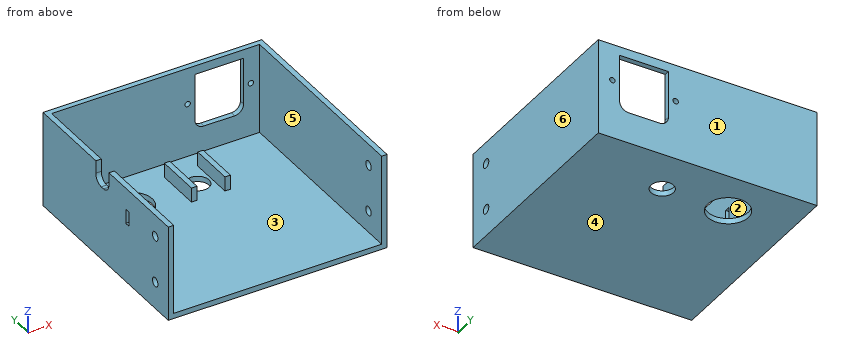
```python
from build123d import *

# Parameters (mm, degrees)
F0_W      = 121
F0_H      = 115
F1_DEPTH  = 3
F3_DEPTH  = 50
F4_R      = 2.5
F5_DEPTH  = 121.001
F6_R      = 11.25
F6_R_2    = 6.25
F7_DEPTH  = 25
F8_W      = 3
F8_H      = 25
F9_DEPTH  = 8
F10_R     = 1.5
F11_DEPTH = 25
F13_DEPTH = 25
F14_R     = 2.5
F14_W     = 3
F14_H     = 8
F15_DEPTH = 25


with BuildPart() as f1:
    # F0 (on Top) → F1 (new body)
    with BuildSketch(Plane.XY):
        with Locations((-4.051243, 22.351279)):
            Rectangle(F0_W, F0_H)
    extrude(amount=F1_DEPTH)

    # F2 (on face) → F3 (join)
    with BuildSketch(Plane.XY.offset(3)):
        Polygon((56.448757, 79.851279), (-64.551243, 79.851279), (-64.551243, -35.148721), (-61.551243, -35.148721), (-61.551243, 76.851279), (53.448757, 76.851279), (53.448757, -35.148721), (56.448757, -35.148721), align=None)
    extrude(amount=F3_DEPTH)

    # F4 (on face) → F5 (cut, through all)
    with BuildSketch(Plane(origin=(-64.551243, 0, 0), x_dir=(0, -1, 0), z_dir=(-1, 0, 0))):
        with Locations((23.148721, 15)):
            Circle(F4_R)
        with Locations((23.148721, 41)):
            Circle(F4_R)
    extrude(amount=-F5_DEPTH, mode=Mode.SUBTRACT)

    # F6 (on face) → F7 (cut)
    with BuildSketch(Plane(origin=(0, 0, 0), x_dir=(1, 0, 0), z_dir=(0, 0, -1))):
        with Locations((-30.708815, -54.351279)):
            Circle(F6_R)
        with Locations((5.693216, -54.351279)):
            Circle(F6_R_2)
    extrude(amount=-F7_DEPTH, mode=Mode.SUBTRACT)

    # F8 (on face) → F9 (join)
    with BuildSketch(Plane.XY.offset(3)):
        with Locations((-3.556784, 54.730202)):
            Rectangle(F8_W, F8_H)
        with Locations((14.943216, 54.730202)):
            Rectangle(F8_W, F8_H)
    extrude(amount=F9_DEPTH)

    # F10 (on face) → F11 (cut)
    with BuildSketch(Plane(origin=(0, 79.851279, 0), x_dir=(-1, 0, 0), z_dir=(0, 1, 0))):
        with BuildLine():
            ThreePointArc((-44.634731, 22.153023), (-43.170264, 18.617489), (-39.634731, 17.153023))
            Line((-39.634731, 17.153023), (-22.634731, 17.153023))
            ThreePointArc((-22.634731, 17.153023), (-19.099197, 18.617489), (-17.634731, 22.153023))
            Line((-17.634731, 22.153023), (-17.634731, 48.153023))
            Line((-17.634731, 48.153023), (-44.634731, 48.153023))
            Line((-44.634731, 48.153023), (-44.634731, 22.153023))
        make_face()
        with Locations((-13.634731, 32.653023)):
            Circle(F10_R)
        with Locations((-48.634731, 32.653023)):
            Circle(F10_R)
    extrude(amount=-F11_DEPTH, mode=Mode.SUBTRACT)

    # F12 (on face) → F13 (cut)
    with BuildSketch(Plane(origin=(-64.551243, 0, 0), x_dir=(0, -1, 0), z_dir=(-1, 0, 0))):
        with BuildLine():
            Line((-19.351279, 62.000753), (-31.351279, 62.000753))
            Line((-31.351279, 62.000753), (-31.351279, 46))
            ThreePointArc((-31.351279, 46), (-29.886813, 42.464466), (-26.351279, 41))
            Line((-26.351279, 41), (-24.351279, 41))
            ThreePointArc((-24.351279, 41), (-20.815745, 42.464466), (-19.351279, 46))
            Line((-19.351279, 46), (-19.351279, 62.000753))
        make_face()
    extrude(amount=-F13_DEPTH, mode=Mode.SUBTRACT)

    # F14 (on face) → F15 (cut)
    with BuildSketch(Plane(origin=(-64.551243, 0, 0), x_dir=(0, -1, 0), z_dir=(-1, 0, 0))):
        with Locations((23.148721, 41)):
            Circle(F14_R)
        with Locations((-2.351279, 37)):
            Rectangle(F14_W, F14_H)
    extrude(amount=-F15_DEPTH, mode=Mode.SUBTRACT)


solid = f1.part
```
Can you work these out from the model? Positions are in its coordinate system, mm. Face numbers are marked on the shaded views. A direction names the side the tool comes from. Coordinates: 2 decimals unless noted, no trailing zeros. Loops run counter-clockwise (first coordinate to the right, second up) from the corner with the lowest first, then second, coordinate; pieces in that order, holes last. Notation, with made-up numbers: M 76.25,23 L 123.25,23 A9 ccw 123.25,31 Z; hole C 31.5,51 d7. An arc over 180 degrees is marked long. Put each result on its own line as item: value. Start each with the question number.
(1) Will these pins go through, and if not, where does the flat tip stop? pin 1 Ø6 at (x, y) = (25.5, 54) entering from +Z; pin 2 Ø1.5 at (x, y) = (-4, 50.5) entering from +Z; pin 3 Ø3.5 at (x, z) = (-3.5, 7) entering from -Y; pin 4 Ø8 at (x, y) = (26.5, 44.5) entering from -Z.
(2) Imagine slicing it at C-C on y = 12.5. List the corners of the cut face in (x, z) for me.
(3) Which directions (+Z, -Z, +X, -X, +Y, -Y) give clear straight access to the entire face, cutting with the end or side of a thin tool? Please do the marked faces 1 and 2.
(4) Imagine slicing it at D-D on x = -7.5. List the corners of the cut face in (y, z) for me.
(5) We'd pull the mould along X, two halves only. Please class the marked faces 3, 4, 5 and 6: +X half, -X half, draft (parallel to the pull), parting line (faces both ways), or undercut.
(6) Imagine slicing it at B-B on x = 31. List the corners of the cut face in (y, z) for me.
(7) Imagine slicing it at A-A on z = 15. List the corners of the cut face in (x, y) for me, and give its area (4 significant figures).
(8) I need wall thicknesses on probe 1 along X at (y, z) = (-9, 24); probe 2 along Z at (x, y) = (-7, -1.5); probe 3 along Y at (x, z) = (45.5, 18). Which ranges of each line are inside material? Lowest first, please.
Worked answers:
1. pin 1: stops at z = 3
1. pin 2: stops at z = 11
1. pin 3: stops at y = 42.23
1. pin 4: stops at z = 0
2. outline: M -64.55,0 L 56.45,0 L 56.45,53 L 53.45,53 L 53.45,3 L -61.55,3 L -61.55,53 L -64.55,53 Z
3. face 1: +Z, -Z, +X, -X, +Y
3. face 2: +Z, -Y
4. outline: M -35.15,0 L 79.85,0 L 79.85,53 L 76.85,53 L 76.85,3 L -35.15,3 Z
5. face 3: undercut
5. face 4: draft
5. face 5: undercut
5. face 6: +X half
6. outline: M -35.15,0 L 79.85,0 L 79.85,17.15 L 76.85,17.15 L 76.85,3 L -35.15,3 Z; M 76.85,48.15 L 79.85,48.15 L 79.85,53 L 76.85,53 Z
7. outline: M -64.55,-35.15 L -61.55,-35.15 L -61.55,-25.65 L -64.55,-25.65 Z; M -64.55,-20.65 L -61.55,-20.65 L -61.55,76.85 L 53.45,76.85 L 53.45,-20.65 L 56.45,-20.65 L 56.45,79.85 L -64.55,79.85 Z; M 53.45,-35.15 L 56.45,-35.15 L 56.45,-25.65 L 53.45,-25.65 Z
7. area: 1,005 mm2
8. probe 1: x = -64.55 to -61.55, 53.45 to 56.45
8. probe 2: z = 0 to 3
8. probe 3: y = 76.85 to 79.85
